from build123d import *

# Parameters (mm, degrees)
F0_R     = 7.5
F1_DEPTH = 30
F0_W     = 7
F0_H     = 42
F2_DEPTH = 6
F3_W     = 7
F3_H     = 42
F4_DEPTH = 24
F6_DEPTH = 18.501


with BuildPart() as f1:
    # F0 (on Top) → F1 (new body)
    with BuildSketch(Plane.XY):
        with BuildLine():
            Line((15, -18), (15, 0))
            ThreePointArc((15, 0), (0, 15), (-15, 0))
            Line((-15, 0), (-15, -18))
            Line((-15, -18), (-3.5, -18))
            Line((-3.5, -18), (3.5, -18))
            Line((3.5, -18), (15, -18))
        make_face()
        Circle(F0_R, mode=Mode.SUBTRACT)
    extrude(amount=F1_DEPTH)

    # F0 (on Top) → F2 (join)
    with BuildSketch(Plane.XY):
        Polygon((15, -51), (15, -18), (3.5, -18), (3.5, -60), (6, -60), align=None)
        with Locations((0, -39)):
            Rectangle(F0_W, F0_H)
        Polygon((-3.5, -18), (-15, -18), (-15, -51), (-6, -60), (-3.5, -60), align=None)
    extrude(amount=F2_DEPTH)

    # F3 (on face) → F4 (join)
    with BuildSketch(Plane.XY.offset(6)):
        with Locations((0, -39)):
            Rectangle(F3_W, F3_H)
    extrude(amount=F4_DEPTH)

    # F5 (on face) → F6 (cut, through all)
    with BuildSketch(Plane.YZ.offset(3.5)):
        Polygon((-60, 30), (-60, 6), (-18, 30), align=None)
    extrude(amount=-F6_DEPTH, mode=Mode.SUBTRACT)


solid = f1.part
Could you check a few things on this model? Use its own coordinates, in mm. A direction names the side the tool comes from. Round coordinates to 2 decimals unless told otherwise and drop trailing zeros. Order: outer loops, then holes, each group sorted by start corner. A loop starts at its lowest first (then second) coordinate and runs counter-clockwise, first axis right, second up.
(1) Please list where these lines run through material, in increasing order: line 1 along X through (y, z) = (-50, 9); line 2 along Y through (x, z) = (5.75, 12.5); line 3 along X through (y, z) = (-2, 3).
Response values:
line 1: x = -3.5 to 3.5
line 2: y = -18 to -4.82, 4.82 to 13.85
line 3: x = -15 to -7.23, 7.23 to 15
(2) Which directions (+Z, -Z, +X, -X, +Y, -Y) give clear straight access to the entire face, cutting with the end or side of a thin tool? Please do faces 1 (the flat face through (3.5, -30, 12)), 2 (the flat face through (-3.5, -30, 12)), 3 (the flat face through (-15, -14, 11)).
Response values:
face 1: +Z, +X, -Y
face 2: +Z, -X, -Y
face 3: +Z, -Z, -X, +Y, -Y
(3) Imagine slicing it at A-A (x = 0). Write out the boundary of the cut face in (y, z), plus the area to 3 significant figures.
Response values:
outline: (-60, 0) - (-7.5, 0) - (-7.5, 30) - (-18, 30) - (-60, 6) - close; (7.5, 0) - (15, 0) - (15, 30) - (7.5, 30) - close
area: 1,300 mm2
(4) Imagine slicing it at D-D (y = -53). Write out the boundary of the cut face in (x, z), plus the area to 3 significant figures.
Response values:
outline: (-13, 0) - (13, 0) - (13, 6) - (3.5, 6) - (3.5, 10) - (-3.5, 10) - (-3.5, 6) - (-13, 6) - close
area: 184 mm2
(5) Imagine slicing it at B-B (z = 21). Write out the boundary of the cut face in (x, y), plus the area to 3 significant figures.
Response values:
outline: (-15, -18) - (-3.5, -18) - (-3.5, -33.75) - (3.5, -33.75) - (3.5, -18) - (15, -18) - (15, 0) arc R15 ccw to (-15, 0) - close; hole circle Ø15 at (0, 0)
area: 827 mm2
(6) If we mould it in two halves opening along Y, with no side actions, what happens to faces 4 (the cylindrical face through (-7.493, 0.33, 14.79)), 5 (the flat face through (-11, -55, 3)), 6 (the cylindrical face through (0, 15, 15)), 7 (the flat face through (0, -9, 30))? For each: released by +Y, released by -Y, zero draft, split by the parting line, or undercut.
Response values:
face 4: undercut
face 5: released by -Y
face 6: released by +Y
face 7: zero draft
(7) I'm going to push flat-ended pins straight in: pin 1 (8 mm diameter, centred on x = -11.5, z = 15, fed in from +Y); pin 2 (3.5 mm diameter, centred on x = -10, y = -37, fed in from +Z); pin 3 (3 mm diameter, centred on x = -11, z = 18, fed in from -Y). Where does each tip first touch, or does it pass through?
Response values:
pin 1: stops at y = 12.99
pin 2: stops at z = 6
pin 3: stops at y = -18
(8) Imagine slicing it at C-C (y = 2). Write out the boundary of the cut face in (x, z).
Response values:
outline: (-14.87, 0) - (-7.23, 0) - (-7.23, 30) - (-14.87, 30) - close; (7.23, 0) - (14.87, 0) - (14.87, 30) - (7.23, 30) - close
